For this review, take the finished solid that the model builds, in its own axes (mm). Face numbers are marked on the shaded views. A direction names the side the tool comes from. Coordinates: 2 decimals unless noted, no trailing zeros. Loops run counter-clockwise (first coordinate to the right, second up) from the corner with the lowest first, then second, coordinate; pieces in that order, holes last. Notation, with made-up numbers: (1.5, 61.5) - (18.5, 61.5) arc R35 cw to (18.5, 98.5) - close; hole circle Ø1 at (-27, 57). An arc over 180 degrees is marked (long way). Answer as a JSON object with one key per item and string values. Group by question number.
Item 1: Clearance check with flat-ended pins moving along their axes: pin 1 (5 mm diameter, centred on y = 7, z = -44, fed in from -X); pin 2 (1.5 mm diameter, centred on x = -124.5, y = -0.5, fed in from -Z); pin 3 (4 mm diameter, centred on x = 120.5, y = -1, fed in from +Z). State where each tip first meets the part, or that it passes through.
Item 2: We need section B-B (x = 114). Give the boundary of the cut face in (y, z), then the cut area to 3 significant figures.
Item 3: Tool access review of the marked faces 1, 2, 3 and 4: name each direction out of +Z, -Z, +X, -X, +Y, -Y from which nothing blocks a thin tool from reaching the whole face with its end or side.
Item 4: We need section A-A (z = 116.5). Give the boundary of the cut face in (x, y), then the cut area to 3 significant figures.
Item 5: To check wall thickness, follow line 1 (Z direction, x = 135, y = 1); line 2 (Y direction, x = 163, z = 188.5); line 3 (Y direction, x = 0, z = -250.5). State the ranges of each line that lie inside material, in increasing order.
Item 6: We need section C-C (y = 8.75). Give the boundary of the cut face in (x, z), then the cut area to 3 significant figures.
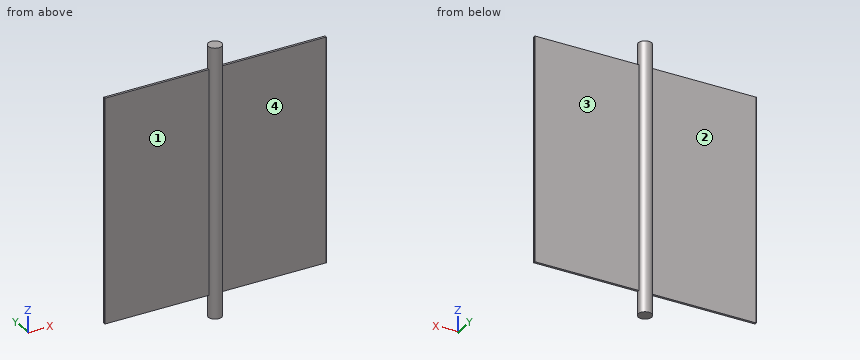
from build123d import *

# Parameters (mm, degrees)
F0_R     = 15
F1_DEPTH = 300
F3_DEPTH = 250


with BuildPart() as f1:
    # F0 (on Top) → F1 (new body, symmetric)
    with BuildSketch(Plane.XY):
        Circle(F0_R)
    extrude(amount=F1_DEPTH, both=True)

    # F2 (on Top) → F3 (join, symmetric)
    with BuildSketch(Plane.XY):
        with BuildLine():
            ThreePointArc((-248, -1.5), (-247.707107, -2.207107), (-247, -2.5))
            Line((-247, -2.5), (247, -2.5))
            ThreePointArc((247, -2.5), (247.707107, -2.207107), (248, -1.5))
            Line((248, -1.5), (248, 1.5))
            ThreePointArc((248, 1.5), (247.707107, 2.207107), (247, 2.5))
            Line((247, 2.5), (-247, 2.5))
            ThreePointArc((-247, 2.5), (-247.707107, 2.207107), (-248, 1.5))
            Line((-248, 1.5), (-248, -1.5))
        make_face()
    extrude(amount=F3_DEPTH, both=True)


solid = f1.part
Check sheet entries:
{
 "1": {"pin 1": "stops at x = -14.31", "pin 2": "stops at z = -250", "pin 3": "stops at z = 250"},
 "2": {"outline": "(-2.5, -250) - (2.5, -250) - (2.5, 250) - (-2.5, 250) - close", "area": "2,500 mm2"},
 "3": {"face 1": "+Z, -Z, -X, -Y", "face 2": "+Z, -Z, -X, +Y", "face 3": "+Z, -Z, +X, +Y", "face 4": "+Z, -Z, +X, -Y"},
 "4": {"outline": "(-248, -1.5) arc R1 ccw to (-247, -2.5) - (-14.79, -2.5) arc R15 ccw to (14.79, -2.5) - (247, -2.5) arc R1 ccw to (248, -1.5) - (248, 1.5) arc R1 ccw to (247, 2.5) - (14.79, 2.5) arc R15 ccw to (-14.79, 2.5) - (-247, 2.5) arc R1 ccw to (-248, 1.5) - close", "area": "3,040 mm2"},
 "5": {"line 1": "z = -250 to 250", "line 2": "y = -2.5 to 2.5", "line 3": "y = -15 to 15"},
 "6": {"outline": "(-12.18, -300) - (12.18, -300) - (12.18, 300) - (-12.18, 300) - close", "area": "14,600 mm2"}
}
